Build history of the part. All positions in model axes, mm. Give positions to 0.01 mm unless a question says otherwise; leave off trailing zeros. Loops run counter-clockwise (first coordinate to the right, second up) from the corner with the lowest first, then second, coordinate; pieces in that order, holes last. Notation, with made-up numbers: (-2.5, 26) - (28.5, 26) arc R13 cw to (28.5, 44) - close; hole circle Ø7 at (30.25, 66). An arc over 180 degrees is marked (long way). Return JSON: item names as keys, results as strings. Group by question number.
1) Slice it at C-C (z = 4.05). List the corners of the cut face in (x, y).
2) Drop flat-ended pins along their axis: pin 1 (0.7 mm diameter, centred on x = 3.5, z = 4, fed in from +Y); pin 2 (3.5 mm diameter, centred on x = -0.5, y = -2, fed in from +Z); pin 3 (0.5 mm diameter, centred on x = 3.5, z = 4, fed in from -Y). Give the stop position or say it passes through.
3) Slice it at A-A (y = 1.5). List the corners of the cut face in (x, z), and give its area (3 significant figures).
4) Slice it at B-B (x = -3). List the corners of the cut face in (y, z), and give its area (3 significant figures).
5) Drill centre line: probe 1 along Z at (x, y) = (-1.75, 2.25). Where is it in solid material? Low to high. Write a range as from..to.
Autodesk Inventor part; units mm, degrees
ref_plane "YZ Plane" through (0, 0, 0) normal (1, 0, 0) x (0, 1, 0)
ref_plane "XZ Plane" through (0, 0, 0) normal (0, 1, 0) x (-1, 0, 0)
ref_plane "XY Plane" through (0, 0, 0) normal (0, 0, 1) x (1, 0, 0)
sketch "草图1" plane through (0, 0, 0) normal (0, 0, 1) x (1, 0, 0)
  line L0 (8.15, -6.1) -> (-8.15, -6.1)
  line L1 (-8.15, -6.1) -> (-8.15, 6.1)
  line L2 (-8.15, 6.1) -> (8.15, 6.1)
  line L3 (8.15, 6.1) -> (8.15, -6.1)
  line L4 (8.15, -6.1) -> (-8.15, 6.1) construction
  line L5 (-8.15, -6.1) -> (8.15, 6.1) construction
  point P0 (0, 0)
  dimension "d0" = 16.3
  dimension "d1" = 12.2
extrude "拉伸1" add sketch "草图1" along normal blind 3.4
sketch "草图2" plane through (0, 0, 3.4) normal (0, 0, 1) x (1, 0, 0)
  line L0 (4.45, 0) -> (4.45, 4.1654) construction
  line L1 (8.15, 6.1) -> (8.15, -6.1) construction
  line L2 (4.45, 3.1034) -> (1.95, 3.1034)
  line L3 (1.95, 3.1034) -> (1.95, -1.7966)
  line L4 (1.95, -1.7966) -> (4.45, -1.7966)
  line L5 (4.45, -1.7966) -> (4.45, 3.1034)
  point P0 (0, 0)
  dimension "d4" = 3.7
  dimension "d5" = 4.9
  dimension "d6" = 2.5
extrude "拉伸2" add sketch "草图2" along normal blind 1
fillet "圆角1" radius 0.1 4 edges at (4.45, 0.6534, 3.4) (3.2, 3.1034, 3.4) (3.2, -1.7966, 3.4) (1.95, 0.6534, 3.4)
properties part number "激光传感器模型" material "氮化硅"
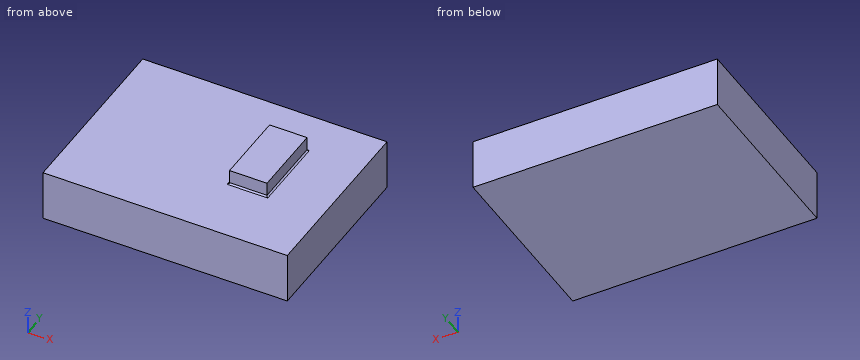
Results:
{
 "1": {"outline": "(1.95, -1.8) - (4.45, -1.8) - (4.45, 3.1) - (1.95, 3.1) - close"},
 "2": {"pin 1": "y = 3.1", "pin 2": "z = 3.4", "pin 3": "y = -1.8"},
 "3": {"outline": "(-8.15, 0) - (8.15, 0) - (8.15, 3.4) - (4.55, 3.4) arc R0.1 cw to (4.45, 3.5) - (4.45, 4.4) - (1.95, 4.4) - (1.95, 3.5) arc R0.1 cw to (1.85, 3.4) - (-8.15, 3.4) - close", "area": "57.9 mm2"},
 "4": {"outline": "(-6.1, 0) - (6.1, 0) - (6.1, 3.4) - (-6.1, 3.4) - close", "area": "41.5 mm2"},
 "5": {"probe 1": "0..3.4"}
}
